Work out the finished part from the listing and answer in its coordinate system (mm). A direction names the side the tool comes from. Coordinates: 2 decimals unless noted, no trailing zeros. Order: outer loops, then holes, each group sorted by start corner. A loop starts at its lowest first (then second) coordinate and runs counter-clockwise, first axis right, second up. Notation, with made-up numbers: M 4,16 L 47,16 A15 cw 47,34 Z; hole C -36,78.5 d3. An arc over 180 degrees is marked long. Write item = value, one per line. Start each with the question number.
Q1. Find section A-A on x = 0. Give the vertices of the cut face in (y, z), and give its area (3 significant figures).
Q2. A tool of negligible diameter and unlimited length cuts with its end or side. For faces 4 (the flat face through (-35.3, 0, 7)), 5 (the flat face through (-14.918, -12.5, 11.6)), 6 (the flat face through (-13, -13, 6)), from which of +Z, -Z, +X, -X, +Y, -Y can it reach the whole face along a straight path? Write none if from no direction.
Q3. Find section C-C on y = 0. Give the vertices of the cut face in (x, z), and give its area (3 significant figures).
Q4. Straight lines are drawn through the part: line 1 along Y through (x, z) = (-25.6, 0.55); line 2 along Y through (x, z) = (-22, 4.75); line 3 along X through (y, z) = (6.5, 6.75). For each, find the intervals that lie inside material, in ascending order.
Q5. This flat-tipped pin is pushed along its axis until it touches: P1, Ø1.1, axis at x = -12.5, y = -12.5, coming from the +Z side. Where does it stop, or does it pass through?
Q6. Determine the mould class of faces 1 (the flat face through (-9.856, -12.5, 11.6)), 2 (the cylindrical face through (-1.73, -7.81, 0.49)), 3 (the flat face through (-13, 13, 6)) for opening direction Y: released by +Y, released by -Y, zero draft, split by the parting line, or undercut.
Q7. Find section B-B on z = 6.5. Give the vertices of the cut face in (x, y), and give its area (3 significant figures).
Q8. Find section D-D on x = -16. Give the vertices of the cut face in (y, z), and give its area (3 significant figures).
```python
from build123d import *

# Parameters (mm, degrees)
SKETCH1_W           = 47
SKETCH1_H           = 26
SKETCH1_W_2         = 45
SKETCH1_H_2         = 24
SKETCH1_R           = 8
BOSS_EXTRUDE1_DEPTH = 1
SKETCH2_W           = 47
SKETCH2_H           = 26
SKETCH2_W_2         = 45
SKETCH2_H_2         = 24
BOSS_EXTRUDE2_DEPTH = 12
CUT_EXTRUDE1_REACH  = 48.505
SKETCH3_W           = 5.061855515
SKETCH3_H           = 3.126915658


with BuildPart() as part:
    # Sketch1 → Boss-Extrude1 (new body)
    # profile 1 of 2: a face of its own
    with BuildSketch(Plane.XY):
        with Locations((-12.8, 0)):
            Rectangle(SKETCH1_W, SKETCH1_H)
        with Locations((-12.8, 0)):
            Rectangle(SKETCH1_W_2, SKETCH1_H_2, mode=Mode.SUBTRACT)
    # profile 2 of 2: a face of its own
    with BuildSketch(Plane.XY):
        with Locations((-12.8, 0)):
            Rectangle(SKETCH1_W_2, SKETCH1_H_2)
        with Locations((-25.6, 0)):
            Circle(SKETCH1_R, mode=Mode.SUBTRACT)
        Circle(SKETCH1_R, mode=Mode.SUBTRACT)
    extrude(amount=BOSS_EXTRUDE1_DEPTH)

    # Sketch2 → Boss-Extrude2 (add)
    with BuildSketch(Plane.XY.offset(1)):
        with Locations((-12.8, 0)):
            Rectangle(SKETCH2_W, SKETCH2_H)
        with Locations((-12.8, 0)):
            Rectangle(SKETCH2_W_2, SKETCH2_H_2, mode=Mode.SUBTRACT)
    extrude(amount=BOSS_EXTRUDE2_DEPTH)

    # Sketch3 → Cut-Extrude1 (cut, up to next)
    with BuildSketch(Plane.XZ.offset(13), mode=Mode.PRIVATE) as cut_extrude1_sk1:
        with Locations((-12.387065936, 11.863457829)):
            Rectangle(SKETCH3_W, SKETCH3_H)
    cut_extrude1_tool1 = extrude(cut_extrude1_sk1.sketch, amount=-CUT_EXTRUDE1_REACH, mode=Mode.PRIVATE) & part.part
    add(cut_extrude1_tool1.solids().sort_by_distance((-12.387066, -13, 11.863458))[0], mode=Mode.SUBTRACT)


solid = part.part
```
Findings below:
q1.outline = M -13,0 L -8,0 L -8,1 L -12,1 L -12,13 L -13,13 Z; M 8,0 L 13,0 L 13,13 L 12,13 L 12,1 L 8,1 Z
q1.area = 34.0 mm^2
q2.face_4 = +Z
q2.face_5 = +Z, -Y
q2.face_6 = +Z, -Z, +X, -X, -Y
q3.outline = M -36.3,0 L -33.6,0 L -33.6,1 L -35.3,1 L -35.3,13 L -36.3,13 Z; M -17.6,0 L -8,0 L -8,1 L -17.6,1 Z; M 8,0 L 10.7,0 L 10.7,13 L 9.7,13 L 9.7,1 L 8,1 Z
q3.area = 39.0 mm^2
q4.line_1 = -13 to -8, 8 to 13
q4.line_2 = -13 to -12, 12 to 13
q4.line_3 = -36.3 to -35.3, 9.7 to 10.7
q5.P1 = 10.3
q6.face_1 = zero draft
q6.face_2 = undercut
q6.face_3 = released by +Y
q7.outline = M -36.3,-13 L 10.7,-13 L 10.7,13 L -36.3,13 Z; hole M -35.3,-12 L 9.7,-12 L 9.7,12 L -35.3,12 Z
q7.area = 142 mm^2
q8.outline = M -13,0 L 13,0 L 13,13 L 12,13 L 12,1 L -12,1 L -12,13 L -13,13 Z
q8.area = 50.0 mm^2
